Design review of the part built by this model. Coordinates are the model's own, in mm. Face numbers are marked on the shaded views. Coordinates: 2 decimals unless noted, no trailing zeros. Loops run counter-clockwise (first coordinate to the right, second up) from the corner with the lowest first, then second, coordinate; pieces in that order, holes last. Notation, with made-up numbers: (21, 72) -> (71, 72) arc R10 ccw to (71, 76) -> close; hole circle Ø5 at (72.5, 72.5). An arc over 180 degrees is marked (long way). One line per item, written item: value. Start each with the question number.
1. Add section B-B on z = 3.5. Write out the cut boundary in (x, y), plus the area to 3 significant figures.
2. Insertion check: pin 1 (7 mm diameter, centred on x = 0, y = 0, fed in from +Z); pin 2 (2 mm diameter, centred on x = 7, z = 4.5, fed in from +Y); pin 3 (4 mm diameter, centred on x = -1.5, z = 9, fed in from +Y); pin 4 (5 mm diameter, centred on x = 0.01, y = -0.02, fed in from -Z). Each pin has a flat end and moves straight along its axis. Give the tip position at first contact, or say it passes through.
3. For probe 1 along Z at (x, y) = (-3, -2.5); probe 2 along Y at (x, z) = (0, 7.25); probe 3 along Y at (x, z) = (1.75, 7.75), list the stretches that pass through material, from the lowest coordinate up.
4. Add section A-A on z = 10.75. Write out the cut boundary in (x, y), plus the area to 3 significant figures.
5. Draft analysis for pull direction X (two halves, no side actions). For the marked faces 1, 2, 3 and 4, state which applies: pulls with the +X half, pulls with the -X half, needs draft (parallel to the pull), parting line crosses it, or undercut.
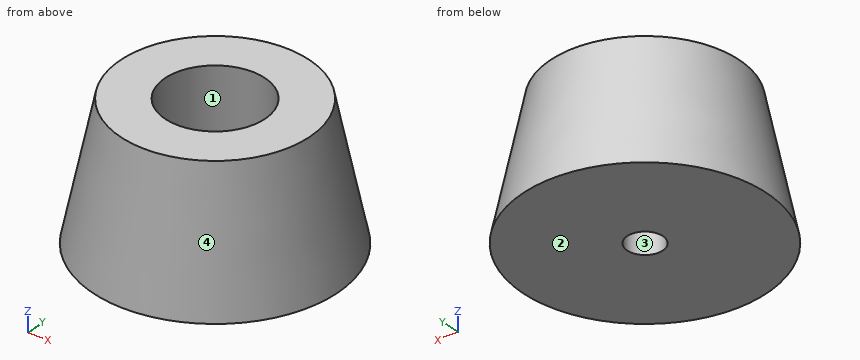
Autodesk Inventor part; units mm, degrees
ref_plane "YZ Plane" through (0, 0, 0) normal (1, 0, 0) x (0, 1, 0)
ref_plane "XZ Plane" through (0, 0, 0) normal (0, 1, 0) x (-1, 0, 0)
sketch "Boceto1" plane through (0, 0, 0) normal (0, 0, 1) x (1, 0, 0)
  circle A0 centre (0, 0) radius 11
  dimension "d0" = 22
ref_plane "Plano de trabajo3" through (0, 0, 5) normal (0, 0, 1) x (1, 0, 0)
sketch "Boceto3" plane through (0, 0, 5) normal (0, 0, 1) x (1, 0, 0)
  circle A0 centre (0, 0) radius 4.5
  circle A1 centre (0, 0) radius 1.5
  dimension "d5" = 9
  dimension "d6" = 3
ref_plane "Plano de trabajo4" through (0, 0, 12) normal (0, 0, 1) x (1, 0, 0)
sketch "Boceto4" plane through (0, 0, 12) normal (0, 0, 1) x (1, 0, 0)
  circle A0 centre (0, 0) radius 8.5
  dimension "d8" = 17
loft "Solevación1" add profiles "Boceto1", "Boceto4"
hole "Agujero3" at (0, 0, 5) direction (0, 0, 1) diameter 9 depth 7
sketch "Boceto5" plane through (0, 0, 5) normal (0, 0, 1) x (1, 0, 0)
  point P0 (0, 0)
  point P1 (0.0057, -0.0188)
hole "Agujero4" at (0.0057, -0.0188, 5) direction (0, 0, -1) diameter 3.2 end through all
properties part number "Patas"
Worked answers:
1. outline: circle Ø20.54 at (0, 0); hole circle Ø3.2 at (0.01, -0.02)
1. area: 323 mm²
2. pin 1: stops at z = 5
2. pin 2: stops at y = 8.12
2. pin 3: stops at y = 9.48
2. pin 4: stops at z = 0
3. probe 1: z = 0 to 5
3. probe 2: y = -9.49 to -4.5, 4.5 to 9.49
3. probe 3: y = -9.22 to -4.15, 4.15 to 9.22
4. outline: circle Ø17.52 at (0, 0); hole circle Ø9 at (0, 0)
4. area: 177 mm²
5. face 1: undercut
5. face 2: needs draft
5. face 3: undercut
5. face 4: parting line crosses it
